CAD build for the part. Positions are in the model's coordinates, mm. Face numbers are marked on the shaded views. A direction names the side the tool comes from. Give positions to 0.01 mm unless a question says otherwise; leave off trailing zeros. Loops run counter-clockwise (first coordinate to the right, second up) from the corner with the lowest first, then second, coordinate; pieces in that order, holes last.
Item 1: Saw through at A-A on x = 62.5. Give the cut face in (y, z).
Item 2: Drop flat-ended pins along their axis: P1, Ø8, axis at x = -6.5, z = 14.5, coming from the +Y side; P2, Ø3, axis at y = -24.5, z = 20.5, coming from the +X side; P3, Ø8, axis at y = -7, z = 20.5, coming from the -X side. Give the stop position or say it passes through.
Item 3: Probe probe 1 along Y at (x, z) = (0, 22); probe 2 along Z at (x, y) = (68, 9); probe 3 along Y at (x, z) = (50.8, 8.75). List the from-to ranges inside material, lowest first.
Item 4: Mould opens along X. For the marked faces 3, 4 and 5 say: released by +X, released by -X, zero draft, split by the parting line, or undercut.
Item 5: Which spindle directions (+Z, -Z, +X, -X, +Y, -Y) get a long thin tool onto all of the face, cutting with end or side? Do the marked faces 1 and 2. Say none if no direction does.
Item 6: Saw through at B-B on z = 26. Give the cut face in (x, y) (1 decimal).
from build123d import *

# Parameters (mm, degrees)
F0_R         = 14.2875
F1_DEPTH     = 41.148
F0_R_2       = 6.35
F2_DEPTH     = 11.176
F4_DEPTH     = 26.67
F6_DEPTH     = 25.4
F7_DEPTH     = 9.398
F8_T4_DEPTH  = 66.4333664876
F8_T9_ANGLE  = 124.391277417
F8_T14_DEPTH = 68.2254329645
F8_T19_ANGLE = 102.7340831682


# Not quite as in the source:
# - a fillet or chamfer that OpenCascade refuses, or shapes differently, is made with other operations: its cross-section is extruded or revolved along the edge and cut away or added


with BuildPart() as f1:
    # F0 (on Top) → F1 (new body)
    with BuildSketch(Plane.XY):
        with BuildLine():
            ThreePointArc((0, -25.4), (17.9605122421, -17.9605122421), (25.4, 0))
            ThreePointArc((25.4, 0), (17.9605122421, 17.9605122421), (0, 25.4))
            ThreePointArc((0, 25.4), (-25.4, 0), (0, -25.4))
        make_face()
        Circle(F0_R, mode=Mode.SUBTRACT)
    extrude(amount=F1_DEPTH)

    # F0 (on Top) → F2 (join)
    with BuildSketch(Plane.XY):
        with BuildLine():
            ThreePointArc((0, 25.4), (17.9605122421, 17.9605122421), (25.4, 0))
            ThreePointArc((25.4, 0), (17.9605122421, -17.9605122421), (0, -25.4))
            Line((0, -25.4), (50.8, -56.9271389808))
            ThreePointArc((50.8, -56.9271389808), (70.1065291687, -57.388260775), (79.8953664876, -40.740937693))
            Line((79.8953664876, -40.740937693), (79.8953664876, 30.8181623129))
            ThreePointArc((79.8953664876, 30.8181623129), (71.3237376894, 46.7274752131), (53.3225332112, 48.3198616445))
            Line((53.3225332112, 48.3198616445), (0, 25.4))
        make_face()
        with Locations((50.8, -40.740937693)):
            Circle(F0_R_2, mode=Mode.SUBTRACT)
        with Locations((53.3225332112, 30.8181623129)):
            Circle(F0_R_2, mode=Mode.SUBTRACT)
    extrude(amount=F2_DEPTH)

    # F3 (on face) → F4 (join)
    with BuildSketch(Plane.XY.offset(11.176)):
        with BuildLine():
            Line((76.5933664876, -9.3715246767), (76.5933664876, 0))
            Line((76.5933664876, 0), (25.4, 0))
            ThreePointArc((25.4, 0), (24.9479609536, -4.77066497), (23.6079335232, -9.3715246767))
            Line((23.6079335232, -9.3715246767), (76.5933664876, -9.3715246767))
        make_face()
    extrude(amount=F4_DEPTH)

    # F5 (on face) → F6 (cut)
    with BuildSketch(Plane.XZ.offset(9.3715246767)):
        Polygon((76.5933664876, 37.846), (30.3995714498, 37.846), (76.5933664876, 11.176), align=None)
    extrude(amount=-F6_DEPTH, mode=Mode.SUBTRACT)

    # F5 (on face) → F7 (join)
    with BuildSketch(Plane.XZ.offset(9.3715246767)):
        Polygon((30.3995714498, 37.846), (25.2215964692, 40.8355052489), (23.6079335232, 40.8355052489), (23.6079335232, 37.846), align=None)
    extrude(amount=-F7_DEPTH)

    # F8: fillet of radius 3.048 on 5 edges, made by hand


with BuildPart() as f8_tool2:
    # F8_s3 → F8_t4 (new body)
    with BuildSketch(Plane.YZ.offset(84.2133664876)):
        with BuildLine():
            ThreePointArc((0, 14.224), (0.8927385309, 12.0687385309), (3.048, 11.176))
            Line((3.048, 11.176), (0, 11.176))
            Line((0, 11.176), (0, 14.224))
        make_face()
    extrude(amount=-F8_T4_DEPTH)

    split(bisect_by=Plane(origin=(23.9876915783, 0, 41.5479005698), x_dir=(0, 1, 0), z_dir=(-0.5, 0, -0.8660254038)), keep=Keep.TOP)


with BuildPart() as f1_1:
    add(f1.part)

    # F8_t1: union F8_tool2
    add(f8_tool2.part)


with BuildPart() as f8_tool7:
    # F8_s8 → F8_t9 (revolve)
    with BuildSketch(Plane(origin=(0, 0, 0), x_dir=(0, 0, 1), z_dir=(-0.2956353345, -0.9553008683, 0))):
        with BuildLine():
            ThreePointArc((14.224, -25.4), (12.0687385309, -26.2927385309), (11.176, -28.448))
            Line((11.176, -28.448), (11.176, -25.4))
            Line((11.176, -25.4), (14.224, -25.4))
        make_face()
    revolve(axis=Axis((0, 0, 11.176), (0, 0, 1)), revolution_arc=F8_T9_ANGLE)

    split(bisect_by=Plane(origin=(-9.2152137271, 21.4389836917, 0), x_dir=(0, 0, 1), z_dir=(0.3948993846, -0.9187243744, 0)), keep=Keep.TOP)


with BuildPart() as f1_2:
    add(f1_1.part)

    # F8_t6: union F8_tool7
    add(f8_tool7.part)


with BuildPart() as f8_tool12:
    # F8_s13 → F8_t14 (new body)
    with BuildSketch(Plane.YZ.offset(15.9879335232)):
        with BuildLine():
            ThreePointArc((-9.3715246767, 14.224), (-10.2642632076, 12.0687385309), (-12.4195246767, 11.176))
            Line((-12.4195246767, 11.176), (-9.3715246767, 11.176))
            Line((-9.3715246767, 11.176), (-9.3715246767, 14.224))
        make_face()
    extrude(amount=F8_T14_DEPTH)

    split(bisect_by=Plane(origin=(23.9876915783, 0, 41.5479005698), x_dir=(0, 1, 0), z_dir=(-0.5, 0, -0.8660254038)), keep=Keep.TOP)


with BuildPart() as f1_3:
    add(f1_2.part)

    # F8_t11: union F8_tool12
    add(f8_tool12.part)


with BuildPart() as f8_tool17:
    # F8_s18 → F8_t19 (revolve)
    with BuildSketch(Plane(origin=(0, 0, 0), x_dir=(0, 0, 1), z_dir=(-0.9553159496, 0.2955865973, 0))):
        with BuildLine():
            ThreePointArc((14.224, -25.4), (12.0687385309, -26.2927385309), (11.176, -28.448))
            Line((11.176, -28.448), (11.176, -25.4))
            Line((11.176, -25.4), (14.224, -25.4))
        make_face()
    revolve(axis=Axis((0, 0, 11.176), (0, 0, 1)), revolution_arc=F8_T19_ANGLE)

    split(bisect_by=Plane(origin=(-11.3803201385, -18.3372256958, 0), x_dir=(0, 0, 1), z_dir=(0.5273158261, 0.8496693589, 0)), keep=Keep.TOP)


with BuildPart() as f1_4:
    add(f1_3.part)

    # F8_t16: union F8_tool17
    add(f8_tool17.part)

    # F8_s21 → F8_t22 (revolve, cut)
    with BuildSketch(Plane.XZ):
        with BuildLine():
            ThreePointArc((17.3355, 41.148), (15.1802385309, 40.2552614691), (14.2875, 38.1))
            Line((14.2875, 38.1), (14.2875, 41.148))
            Line((14.2875, 41.148), (17.3355, 41.148))
        make_face()
    revolve(axis=Axis((0, 0, 41.148), (0, 0, 1)), mode=Mode.SUBTRACT)


solid = f1_4.part
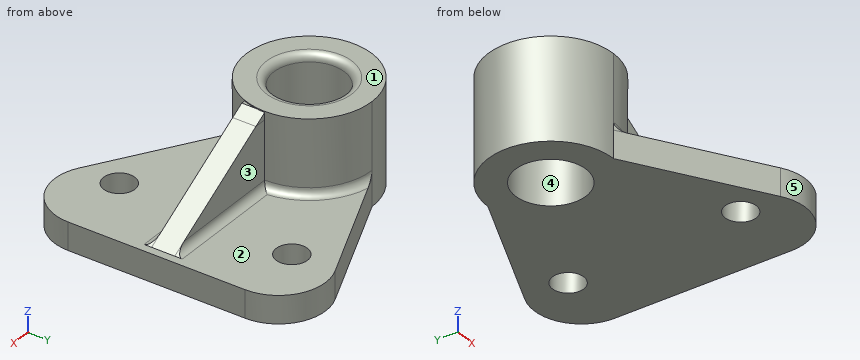
Results below:
1. outline: (-59.72, 0) - (49.8, 0) - (49.8, 11.18) - (3.05, 11.18) arc R3.05 cw to (0, 14.22) - (0, 19.31) - (-9.37, 19.31) - (-9.37, 14.22) arc R3.05 cw to (-12.42, 11.18) - (-59.72, 11.18) - close
2. P1: stops at y = 25.28
2. P2: stops at x = 10.78
2. P3: stops at x = -25.22
3. probe 1: y = -25.4 to -14.29, 14.29 to 25.4
3. probe 2: z = 0 to 11.18
3. probe 3: y = -56.93 to -47.09, -34.39 to 24.99, 36.65 to 47.24
4. face 3: zero draft
4. face 4: undercut
4. face 5: split by the parting line
5. face 1: +Z, +X, -X, +Y, -Y
5. face 2: +Z, +X
6. outline: (23.6, -9.4) - (50.9, -9.4) - (50.9, 0) - (25.4, 0) arc R25.4 ccw (long way) to start; hole circle Ø28.6 at (0, 0)
